Autodesk Inventor part; units mm, degrees
ref_plane "YZ Plane" through (0, 0, 0) normal (1, 0, 0) x (0, 1, 0)
ref_plane "XZ Plane" through (0, 0, 0) normal (0, 1, 0) x (-1, 0, 0)
ref_plane "XY Plane" through (0, 0, 0) normal (0, 0, 1) x (1, 0, 0)
sketch "Skizze1" plane through (0, 0, 0) normal (0, 1, 0) x (-1, 0, 0)
  arc A0 (-0.4888, 25.4953) -> (-25.5, 0) centre (0, 0) ccw
  arc A1 (-7.4888, 29.9259) -> (-30.8486, 0) centre (0, 0) ccw
  line L0 (-0.4888, 25.4953) -> (-0.4888, 39.9953)
  line L1 (-0.4888, 39.9953) -> (-7.4888, 39.9953)
  line L2 (-7.4888, 39.9953) -> (-7.4888, 29.9259)
  line L3 (0, 0) -> (-16.7346, 0) construction
  arc A2 (-25.5, 0) -> (-0.4888, -25.4953) centre (0, 0) ccw
  arc A3 (-30.8486, 0) -> (-7.4888, -29.9259) centre (0, 0) ccw
  line L4 (-0.4888, -25.4953) -> (-0.4888, -39.9953)
  line L5 (-0.4888, -39.9953) -> (-7.4888, -39.9953)
  line L6 (-7.4888, -39.9953) -> (-7.4888, -29.9259)
  dimension "d5" = 14.5
  dimension "d6" = 25.5
  dimension "d8" = 10.0694
  dimension "d9" = 7
  dimension "d52" = 30.8486
extrude "Extrusion1" add sketch "Skizze1" along normal blind 20
sketch "Skizze2" plane through (0.4888, 0, 25.4953) normal (-1, 0, 0) x (0, 0, 1)
  line L0 (14.5, 0) -> (14.5, 20)
  line L1 (14.5, 10) -> (-98.2028, 10) construction
  line L2 (0, 20) -> (14.5, 20)
  line L3 (-65.4906, 0) -> (-65.4906, 20)
  point P0 (-25.4953, 0)
  point P1 (9.5, 10)
  point P2 (-60.4906, 10)
  dimension "d12" = 10
  dimension "d13" = 5
  dimension "d14" = 5
hole "Bohrung1" at (0.4888, 10, 34.9953) at (0.4888, 10, -34.9953) direction (1, 0, 0) diameter 3 end through all
ref_plane "Arbeitsebene1" through (30.8486, 20, 0) normal (1, 0, 0) x (0, 1, 0)
sketch "Skizze3" plane through (30.8486, 20, 0) normal (1, 0, 0) x (0, 1, 0)
  line L0 (0, 25.4953) -> (0, -25.4953)
  line L1 (0, 15) -> (-20, 15)
  line L2 (-20, 15) -> (-20, -15)
  line L3 (-20, -15) -> (0, -15)
  line L4 (0, -15) -> (0, 15)
  point P0 (-20, 0)
  dimension "d28" = 20
  dimension "d30" = 15
  dimension "d31" = 15
extrude "Extrusion2" cut sketch "Skizze3" against normal blind 1
sketch "Skizze4" plane through (30.8486, 20, 0) normal (1, 0, 0) x (0, 1, 0)
  line L0 (0, -7.7908) -> (-20, -7.7908) construction
  line L1 (-10, -7.7908) -> (-10, 7.7908) construction
  line L2 (-20, 7.7908) -> (0, 7.7908) construction
  line L3 (-20, 0) -> (0, 0) construction
  line L4 (0, 25.4953) -> (0, -25.4953) construction
  point P0 (-10, -5)
  point P1 (-10, 5)
  dimension "d49" = 5
  dimension "d50" = 5
hole "Bohrung2" at (30.8486, 10, -5) at (30.8486, 10, 5) direction (-1, 0, 0) diameter 3 end through all
chamfer "Fase2" distance 1 angle 45 1 edges at (25.2587, 9.9941, -3.5)
chamfer "Fase3" distance 1 angle 45 1 edges at (24.6577, 9.994, 6.5)
properties part number "spannringe"
Model file for the job. Use its own axes, mm. A direction names the side the tool comes from. Give positions to 0.01 mm unless a question says otherwise; leave off trailing zeros. Loops run counter-clockwise (first coordinate to the right, second up) from the corner with the lowest first, then second, coordinate; pieces in that order, holes last.
1) Saw through at A-A (x = 8.25). Write the cut outline in (y, z).
2) Pull direction Z, two halves, no side cores. Call faces 5 (the cylindrical face through (18.396, 9.86, 17.659)), 6 (the flat face through (0.489, 10, 33)), 7 (the cylindrical face through (21.538, 9.86, -22.085)): +Z half, -Z half, draft (parallel to the pull), parting line (faces both ways), or undercut.
3) Tool access for faces 1 (the flat face through (7.489, 8, 35)), 2 (the cylindrical face through (4.038, 10.913, 33.805)), 3 (the cylindrical face through (18.01, 9.86, -18.05)), 4 (the flat face through (7.489, 8, -35)): list every direction of +Z, -Z, +X, -X, +Y, -Y with a clear straight run to the whole face (end or side of a thin tool).
4) Saw through at C-C (y = 10). Count the separate pieces of the cut face and the enclosed holes in it, plus the area to 3 significant figures.
5) Saw through at B-B (y = 2). Write the cut outline in (x, z), plus the area to 3 significant figures.
6) Flat gauge pins, fed straight in: pin 1 Ø5 at (y, z) = (7, -32.5) entering from +X; pin 2 Ø1 at (y, z) = (4, 13) entering from -X; pin 3 Ø1.5 at (y, z) = (15.5, -22.5) entering from -X. Where does each tip first touch, or does it go through?
7) Saw through at D-D (z = 19). Write the cut outline in (x, y).
8) Wall check: line 1 (Z direction, x = 2.75, y = 10); line 2 (Z direction, x = 4, y = 10.5); line 3 (X direction, y = 17.75, z = 33). Give the ranges that are in metal, low to high.
Answer block:
1. outline: (0, -29.73) - (20, -29.73) - (20, -24.13) - (0, -24.13) - close; (0, 24.13) - (20, 24.13) - (20, 29.73) - (0, 29.73) - close
2. face 5: undercut
2. face 6: draft
2. face 7: -Z half
3. face 1: +Z, +X, +Y, -Y
3. face 2: +X, -X
3. face 3: -X, +Y, -Y
3. face 4: -Z, +X, +Y, -Y
4. separate pieces: 5
4. enclosed holes: 0
4. area: 517 mm2
5. outline: (0.49, -40) - (7.49, -40) - (7.49, -29.93) arc R30.85 ccw to (29.85, -7.79) - (29.85, 7.79) arc R30.85 ccw to (7.49, 29.93) - (7.49, 40) - (0.49, 40) - (0.49, 25.5) arc R25.5 cw to (25.5, 0) arc R25.5 cw to (0.49, -25.5) - close
5. area: 590 mm2
6. pin 1: stops at x = 7.49
6. pin 2: stops at x = 21.63
6. pin 3: stops at x = 10.47
7. outline: (17.01, 0) - (24.3, 0) - (24.3, 20) - (17.01, 20) - close
8. line 1: z = -40 to -36.5, -33.5 to -25.35, 25.35 to 33.5, 36.5 to 40
8. line 2: z = -40 to -36.41, -33.58 to -25.18, 25.18 to 33.58, 36.41 to 40
8. line 3: x = 0.49 to 7.49
